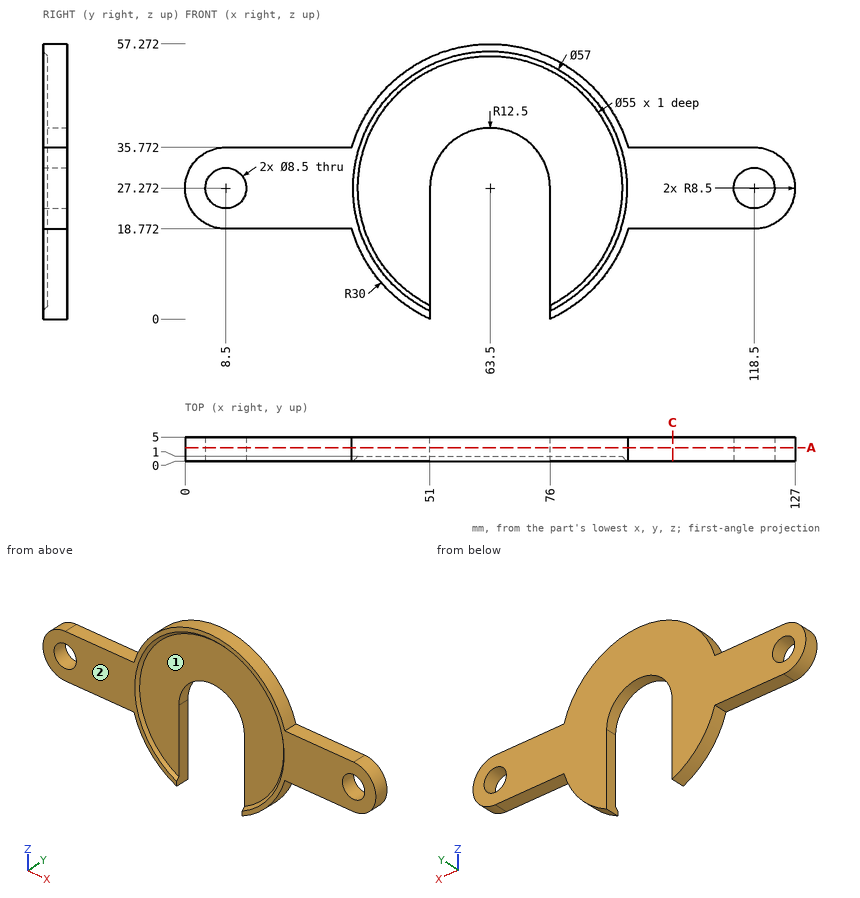
Print and shaded views of the part. All mm, measured from the part's lowest x, y and z. Coordinates: 2 decimals unless noted, no trailing zeros. Write each loop counter-clockwise with the first axis right and the second up, starting at its lowest first coordinate (ties: lowest second). Pieces come first, ordered by that corner, then holes.
(1) Two-plate mould, pull along Z, no slides. Class the marked faces 1 and 2: +Z half, -Z half, draft (parallel to the pull), parting line (faces both ways), or undercut.
(2) Flat gauge pins, fed straight in: pin 1 (6 mm diameter, centred on x = 73, z = 46, fed in from -Y); pin 2 (2.5 mm diameter, centred on x = 107.5, y = 2.5, fed in from -Z); pin 3 (1.5 mm diameter, centred on y = 3.5, z = 16, fed in from +X); pin 4 (7 mm diameter, centred on x = 8.5, z = 27.27, fed in from +Y). Where does each tip first touch, or does it go through?
(3) Cut at A-A, the plane y = 2.8. List the corners of the cut face in (x, z).
(4) Cut at C-C, the plane x = 101.5. List the corners of the cut face in (y, z), and give its area (3 significant figures).
(5) Drill centre lines: probe 1 along X at (y, z) = (2.55, 29); probe 2 along X at (y, z) = (1.1, 28); probe 3 along Z at (x, y) = (24.5, 2.5). Where is each one in solid material? Low to high.
Geometry says:
1. face 1: undercut
1. face 2: draft
2. pin 1: stops at y = 1
2. pin 2: stops at z = 18.77
2. pin 3: stops at x = 91.59
2. pin 4: passes through
3. outline: (8.5, 18.77) - (34.73, 18.77) arc R30 ccw to (51, 0) - (51, 27.27) arc R12.5 cw to (76, 27.27) - (76, 0) arc R30 ccw to (92.27, 18.77) - (118.5, 18.77) arc R8.5 ccw to (118.5, 35.77) - (92.27, 35.77) arc R30 ccw to (34.73, 35.77) - (8.5, 35.77) arc R8.5 ccw to start; hole circle Ø8.5 at (8.5, 27.27); hole circle Ø8.5 at (118.5, 27.27)
4. outline: (0, 18.77) - (5, 18.77) - (5, 35.77) - (0, 35.77) - close
4. area: 85.0 mm2
5. probe 1: x = 0.18 to 4.62, 12.38 to 51.12, 75.88 to 114.62, 122.38 to 126.82
5. probe 2: x = 0.03 to 4.31, 12.69 to 51.02, 75.98 to 114.31, 122.69 to 126.97
5. probe 3: z = 18.77 to 35.77
